Build history of the part. All positions in model axes, mm. Give positions to 0.01 mm unless a question says otherwise; leave off trailing zeros. Order: outer loops, then holes, each group sorted by start corner. A loop starts at its lowest first (then second) coordinate and runs counter-clockwise, first axis right, second up. Notation, with made-up numbers: (-27, -16.75) -> (8, -16.75) arc R19 ccw to (8, 10.25) -> close; hole circle Ø11 at (27, 33). An arc over 180 degrees is marked (long way). Write item = value, one per line. Start each with the question number.
from build123d import *

# Parameters (mm, degrees)
SKETCH1_W           = 107.95
SKETCH1_H           = 31.75
SKETCH1_H_2         = 53.975
BOSS_EXTRUDE1_DEPTH = 6.35
SKETCH11_R          = 2.54
CUT_EXTRUDE2_DEPTH  = 7.62
SKETCH12_W          = 11.43
SKETCH12_H          = 1.016
CUT_EXTRUDE3_DEPTH  = 7.62
SKETCH13_R          = 3.175
CUT_EXTRUDE4_DEPTH  = 7.62


with BuildPart() as part:
    # Sketch1 → Boss-Extrude1 (new body)
    with BuildSketch(Plane.XY):
        with Locations((0, 15.875)):
            Rectangle(SKETCH1_W, SKETCH1_H)
        with Locations((0, -26.9875)):
            Rectangle(SKETCH1_W, SKETCH1_H_2)
    extrude(amount=BOSS_EXTRUDE1_DEPTH)

    # Sketch11 → Cut-Extrude2 (cut)
    with BuildSketch(Plane(origin=(0, 0, 0), x_dir=(-1, 0, 0), z_dir=(0, 0, -1))):
        with Locations((23.622, -23.622)):
            Circle(SKETCH11_R)
        with Locations((-23.622, -23.622)):
            Circle(SKETCH11_R)
        with Locations((-23.622, 23.622)):
            Circle(SKETCH11_R)
        with Locations((23.622, 23.622)):
            Circle(SKETCH11_R)
    extrude(amount=-CUT_EXTRUDE2_DEPTH, mode=Mode.SUBTRACT)

    # Sketch12 → Cut-Extrude3 (cut)
    with BuildSketch(Plane(origin=(0, 0, 0), x_dir=(-1, 0, 0), z_dir=(0, 0, -1))):
        with BuildLine():
            ThreePointArc((-25.027545804, -18.46622785), (-27.542017518, -17.424699564), (-28.583545804, -14.91022785))
            Line((-28.583545804, -14.91022785), (-28.583545804, 15.26497215))
            ThreePointArc((-28.583545804, 15.26497215), (-27.542017518, 17.779443863), (-25.027545804, 18.82097215))
            Line((-25.027545804, 18.82097215), (-23.630545804, 18.82097215))
            ThreePointArc((-23.630545804, 18.82097215), (-20.110285404, 20.27911175), (-18.652145804, 23.79937215))
            Line((-18.652145804, 23.79937215), (-18.652145804, 25.19637215))
            ThreePointArc((-18.652145804, 25.19637215), (-17.610617518, 27.710843863), (-15.096145804, 28.75237215))
            Line((-15.096145804, 28.75237215), (15.079054196, 28.75237215))
            ThreePointArc((15.079054196, 28.75237215), (17.59352591, 27.710843863), (18.635054196, 25.19637215))
            Line((18.635054196, 25.19637215), (18.635054196, 23.79937215))
            ThreePointArc((18.635054196, 23.79937215), (20.093193797, 20.27911175), (23.613454196, 18.82097215))
            Line((23.613454196, 18.82097215), (25.010454196, 18.82097215))
            ThreePointArc((25.010454196, 18.82097215), (27.52492591, 17.779443863), (28.566454196, 15.26497215))
            Line((28.566454196, 15.26497215), (28.566454196, -14.91022785))
            ThreePointArc((28.566454196, -14.91022785), (27.52492591, -17.424699564), (25.010454196, -18.46622785))
            Line((25.010454196, -18.46622785), (23.613454196, -18.46622785))
            ThreePointArc((23.613454196, -18.46622785), (20.093193797, -19.924367451), (18.635054196, -23.44462785))
            Line((18.635054196, -23.44462785), (18.635054196, -24.84162785))
            ThreePointArc((18.635054196, -24.84162785), (17.59352591, -27.356099564), (15.079054196, -28.39762785))
            Line((15.079054196, -28.39762785), (-15.096145804, -28.39762785))
            ThreePointArc((-15.096145804, -28.39762785), (-17.610617518, -27.356099564), (-18.652145804, -24.84162785))
            Line((-18.652145804, -24.84162785), (-18.652145804, -23.44462785))
            ThreePointArc((-18.652145804, -23.44462785), (-20.110285404, -19.924367451), (-23.630545804, -18.46622785))
            Line((-23.630545804, -18.46622785), (-25.027545804, -18.46622785))
        make_face()
        with Locations((-0.008545804, -28.90562785)):
            Rectangle(SKETCH12_W, SKETCH12_H)
    extrude(amount=-CUT_EXTRUDE3_DEPTH, mode=Mode.SUBTRACT)

    # Sketch13 → Cut-Extrude4 (cut)
    with BuildSketch(Plane(origin=(0, 0, 0), x_dir=(-1, 0, 0), z_dir=(0, 0, -1))):
        with Locations((-41.283545804, 16.05237215)):
            Circle(SKETCH13_R)
        with Locations((-41.283545804, -41.275)):
            Circle(SKETCH13_R)
        with Locations(Location((41.283545804, -41.275, 0), (0, 0, 180))):
            Circle(SKETCH13_R)
        with Locations(Location((41.283545804, 16.05237215, 0), (0, 0, 180))):
            Circle(SKETCH13_R)
    extrude(amount=-CUT_EXTRUDE4_DEPTH, mode=Mode.SUBTRACT)


solid = part.part
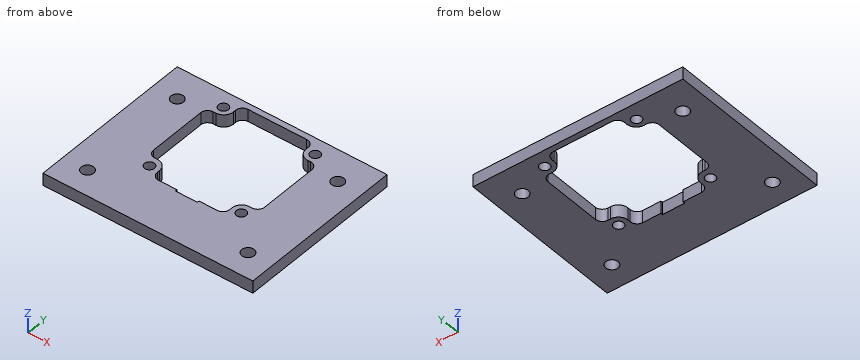
(1) Cut at C-C, the plane z = 4.5. Give the number of separate pieces and of enclosed holes in the cut face, plus the area to 3 significant figures.
(2) Flat gauge pin, fed straight in: P1, Ø3, axis at x = 23.622, y = -23.622, coming from the -Z side. Where does the tip first touch, or does it go through?
(3) Cut at B-B, the plane x = -9.5. Give the cut face in (y, z) (3 decimals).
(4) Cut at A-A, the plane y = -11. Give the cut face in (x, z) (3 decimals), plus the area to 3 significant figures.
(5) Wall check: line 1 (Y direction, x = -23.5, z = 1) (3 decimals); line 2 (X direction, y = -23.5, z = 5) (3 decimals); line 3 (Y direction, x = -1, z = 4) (3 decimals). Give the ranges that are in metal, low to high. Write a range as [from, to].
Results:
q1.separate_pieces = 1
q1.enclosed_holes = 9
q1.area = 6,160 mm2
q2.P1 = through
q3.outline = (-53.975, 0) -> (-28.398, 0) -> (-28.398, 6.35) -> (-53.975, 6.35) -> close; (28.752, 0) -> (31.75, 0) -> (31.75, 6.35) -> (28.752, 6.35) -> close
q4.outline = (-53.975, 0) -> (-28.566, 0) -> (-28.566, 6.35) -> (-53.975, 6.35) -> close; (28.584, 0) -> (53.975, 0) -> (53.975, 6.35) -> (28.584, 6.35) -> close
q4.area = 323 mm2
q5.line_1 = [-53.975, -26.159], [-21.085, -18.468], [18.822, 21.085], [26.159, 31.75]
q5.line_2 = [-53.975, -26.159], [-21.085, -18.635], [18.652, 21.085], [26.159, 53.975]
q5.line_3 = [-53.975, -29.414], [28.752, 31.75]
